Read the model definition and answer for the solid it produces. Units are mm, in the model's axes. Round coordinates to 2 decimals unless told otherwise and drop trailing zeros. Loops run counter-clockwise (first coordinate to the right, second up) from the corner with the lowest first, then second, coordinate; pieces in that order, holes last. Notation, with made-up numbers: (68, 70) - (127, 70) arc R18 ccw to (127, 83) - close; hole circle Ø8 at (43, 40.5). An arc over 180 degrees is marked (long way). Use CSV: the item, a comma, the result in double quotes. Start each with the question number.
1. Find section A-A (y = 0). Give the vertices of the cut face in (x, z).
2. Consider line 1 along Y through (x, z) = (0, 1.5); line 2 along Y through (x, z) = (-1, 0.95); line 3 along X through (y, z) = (27.5, 1.45). Determine where each line is inside the solid, lowest interval first.
3. Given pin 1 Ø6.5 at (x, y) = (0, 55) entering from +Z; pin 2 Ø17.5 at (x, y) = (-47.63, 27.5) entering from -Z; pin 3 Ø12.5 at (x, y) = (-47.63, -27.5) entering from -Z; pin 4 Ø3 at (x, y) = (-40.5, 25.5) entering from -Z, each flat-ended and moving along its own axis, determine where each tip first touches the part or whether it passes through.
4. Find section C-C (z = -1.85). Give the vertices of the cut face in (x, y) (3 decimals).
5. Determine the mould class of faces 1 (the flat face through (-18, 18, 3)), 2 (the cylindrical face through (-9.764, 74.362, 0.042)), 3 (the cylindrical face through (-42.4, 29.2, 1.8)) for opening direction Y: +Y half, -Y half, draft (parallel to the pull), parting line (faces both ways), or undercut.
6. Find section B-B (x = 0). Give the vertices of the cut face in (y, z) (3 decimals).
7. Find section D-D (y = -27.5). Give the vertices of the cut face in (x, z) (3 decimals).
from build123d import *

# Parameters (mm, degrees)
SKETCH_1_R                  = 75
SKETCH_1_R_2                = 25
SKETCH_1_R_3                = 5.5
EXTRUDE_1_DEPTH             = 3
HOLE_WIZARD_M81_D           = 9
HOLE_WIZARD_M81_DEPTH       = 17
HOLE_WIZARD_M81_CSINK_D     = 18.25
HOLE_WIZARD_M81_CSINK_ANGLE = 90
HOLE_WIZARD_M81_TIP         = 2.703872786


with BuildPart() as part:
    # Эскиз1 → Бобышка-Вытянуть1 (new, symmetric)
    with BuildSketch(Plane.XY):
        Circle(SKETCH_1_R)
        Circle(SKETCH_1_R_2, mode=Mode.SUBTRACT)
        with Locations((0, 55)):
            Circle(SKETCH_1_R_3, mode=Mode.SUBTRACT)
        with Locations((47.631397208, 27.5)):
            Circle(SKETCH_1_R_3, mode=Mode.SUBTRACT)
        with Locations((47.631397208, -27.5)):
            Circle(SKETCH_1_R_3, mode=Mode.SUBTRACT)
        with Locations((0, -55)):
            Circle(SKETCH_1_R_3, mode=Mode.SUBTRACT)
        with Locations((-47.631397208, -27.5)):
            Circle(SKETCH_1_R_3, mode=Mode.SUBTRACT)
        with Locations((-47.631397208, 27.5)):
            Circle(SKETCH_1_R_3, mode=Mode.SUBTRACT)
    extrude(amount=EXTRUDE_1_DEPTH, both=True)

    # Зенковка для винта с потайной головкой и внутренним шестигранником M81
    with Locations(Plane(origin=(0, 0, -3), x_dir=(-1, 0, 0), z_dir=(0, 0, -1))):
        with Locations((0, 55), (47.631397208, 27.5), (47.631397208, -27.5), (0, -55), (-47.631397208, -27.5), (-47.631397208, 27.5)):
            CounterSinkHole(HOLE_WIZARD_M81_D / 2, HOLE_WIZARD_M81_CSINK_D / 2, depth=HOLE_WIZARD_M81_DEPTH, counter_sink_angle=HOLE_WIZARD_M81_CSINK_ANGLE)
            with Locations((0, 0, -(HOLE_WIZARD_M81_DEPTH + HOLE_WIZARD_M81_TIP / 2))):  # 118° drill point
                Cone(0, HOLE_WIZARD_M81_D / 2, HOLE_WIZARD_M81_TIP, mode=Mode.SUBTRACT)


solid = part.part
Filled sheet:
1,outline,"(-75, -3) - (-25, -3) - (-25, 3) - (-75, 3) - close; (25, -3) - (75, -3) - (75, 3) - (25, 3) - close"
2,line 1,"y = -75 to -60.5, -49.5 to -25, 25 to 49.5, 60.5 to 75"
2,line 2,"y = -74.99 to -60.41, -49.59 to -24.98, 24.98 to 49.59, 60.41 to 74.99"
2,line 3,"x = -69.78 to -53.13, -42.13 to 42.13, 53.13 to 69.78"
3,pin 1,"passes through"
3,pin 2,"stops at z = -2.63"
3,pin 3,"stops at z = -0.13"
3,pin 4,"stops at z = -2.78"
4,outline,"circle Ø150 at (0, 0); hole circle Ø15.95 at (-47.631, -27.5); hole circle Ø15.95 at (-47.631, 27.5); hole circle Ø50 at (0, 0); hole circle Ø15.95 at (0, -55); hole circle Ø15.95 at (0, 55); hole circle Ø15.95 at (47.631, -27.5); hole circle Ø15.95 at (47.631, 27.5)"
5,face 1,"draft"
5,face 2,"parting line"
5,face 3,"undercut"
6,outline,"(-75, -3) - (-64.125, -3) - (-60.5, 0.625) - (-60.5, 3) - (-75, 3) - close; (-49.5, 0.625) - (-45.875, -3) - (-25, -3) - (-25, 3) - (-49.5, 3) - close; (25, -3) - (45.875, -3) - (49.5, 0.625) - (49.5, 3) - (25, 3) - close; (60.5, 0.625) - (64.125, -3) - (75, -3) - (75, 3) - (60.5, 3) - close"
7,outline,"(-69.776, -3) - (-56.756, -3) - (-53.131, 0.625) - (-53.131, 3) - (-69.776, 3) - close; (-42.131, 0.625) - (-38.506, -3) - (38.506, -3) - (42.131, 0.625) - (42.131, 3) - (-42.131, 3) - close; (53.131, 0.625) - (56.756, -3) - (69.776, -3) - (69.776, 3) - (53.131, 3) - close"
